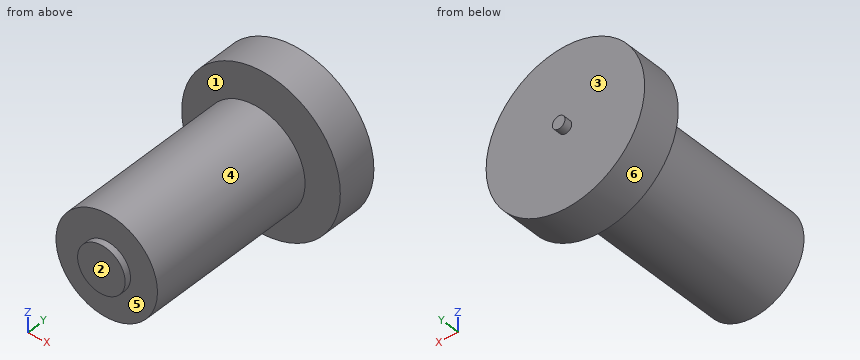
```python
from build123d import *

# Parameters (mm, degrees)
SKETCH1_R           = 32
BOSS_EXTRUDE1_DEPTH = 110
SKETCH2_R           = 5
BOSS_EXTRUDE2_DEPTH = 5
SKETCH3_R           = 50
BOSS_EXTRUDE3_DEPTH = 25
SKETCH4_R           = 4
BOSS_EXTRUDE4_DEPTH = 5
SKETCH5_R           = 15
BOSS_EXTRUDE5_DEPTH = 4


with BuildPart() as part:
    # Sketch1 → Boss-Extrude1 (new body)
    with BuildSketch(Plane(origin=(0, 0, 0), x_dir=(1, 0, 0), z_dir=(0, 1, 0))):
        Circle(SKETCH1_R)
    extrude(amount=BOSS_EXTRUDE1_DEPTH)

    # Sketch2 → Boss-Extrude2 (add)
    with BuildSketch(Plane(origin=(0, 110, 0), x_dir=(1, 0, 0), z_dir=(0, 1, 0))):
        Circle(SKETCH2_R)
    extrude(amount=BOSS_EXTRUDE2_DEPTH)

    # Sketch3 → Boss-Extrude3 (add)
    with BuildSketch(Plane(origin=(0, 115, 0), x_dir=(1, 0, 0), z_dir=(0, 1, 0))):
        Circle(SKETCH3_R)
    extrude(amount=BOSS_EXTRUDE3_DEPTH)

    # Sketch4 → Boss-Extrude4 (add)
    with BuildSketch(Plane(origin=(0, 140, 0), x_dir=(1, 0, 0), z_dir=(0, 1, 0))):
        Circle(SKETCH4_R)
    extrude(amount=BOSS_EXTRUDE4_DEPTH)

    # Sketch5 → Boss-Extrude5 (add)
    with BuildSketch(Plane.XZ):
        Circle(SKETCH5_R)
    extrude(amount=BOSS_EXTRUDE5_DEPTH)


solid = part.part
```
CAD build for the part. Positions are in the model's coordinates, mm. Face numbers are marked on the shaded views. A direction names the side the tool comes from. Coordinates: 2 decimals unless noted, no trailing zeros. Order: outer loops, then holes, each group sorted by start corner. A loop starts at its lowest first (then second) coordinate and runs counter-clockwise, first axis right, second up. Notation, with made-up numbers: M 18.5,-36.75 L 27.5,-36.75 A21 cw 27.5,-17.75 Z; hole C 78,-34.5 d2. An arc over 180 degrees is marked long. Write each question's results on one line, items separated by ' | '. Start each with the question number.
Q1. Drill centre lines: probe 1 along Y at (x, z) = (4.5, 28.5); probe 2 along Y at (x, z) = (-0.5, -43); probe 3 along Y at (x, z) = (5, -7.5). Where is each one in solid material? Low to high. Write a range as from..to.
Q2. Cut at B-B (z = 0). List the corners of the cut face in (x, y), then the cut area to 3 significant figures.
Q3. Cut at A-A (x = 12). List the corners of the cut face in (y, z).
Q4. Cut at C-C (z = 21). List the corners of the cut face in (x, y), then the cut area to 3 significant figures.
Q5. Which spindle directions (+Z, -Z, +X, -X, +Y, -Y) get a long thin tool onto all of the face, cutting with end or side? Do the marked faces 5 and 6. Say none if no direction does.
Q6. Flat gauge pins, fed straight in: P1, Ø8, axis at x = 34, z = 24, coming from the -Y side; P2, Ø1.5, axis at x = -39, z = 30, coming from the +Y side; P3, Ø3, axis at x = -0.5, z = -30, coming from the -Y side. Where does each tip first touch, or does it go through?
Q7. Cut at D-D (x = 0). List the corners of the cut face in (y, z).
Q8. Pull direction Y, two halves, no side cores. Call the marked faces 1, 2, 3 and 4: +Y half, -Y half, draft (parallel to the pull), parting line (faces both ways), or undercut.
Found:
1) probe 1: 0..110, 115..140 | probe 2: 115..140 | probe 3: -4..110, 115..140
2) outline: M -50,115 L -5,115 L -5,110 L -32,110 L -32,0 L -15,0 L -15,-4 L 15,-4 L 15,0 L 32,0 L 32,110 L 5,110 L 5,115 L 50,115 L 50,140 L 4,140 L 4,145 L -4,145 L -4,140 L -50,140 Z | area: 9,750 mm²
3) outline: M -4,-9 L 0,-9 L 0,-29.66 L 110,-29.66 L 110,29.66 L 0,29.66 L 0,9 L -4,9 Z; M 115,-48.54 L 140,-48.54 L 140,48.54 L 115,48.54 Z
4) outline: M -45.38,115 L 45.38,115 L 45.38,140 L -45.38,140 Z; M -24.15,0 L 24.15,0 L 24.15,110 L -24.15,110 Z | area: 7,580 mm²
5) face 5: -Y | face 6: +Y, -Y
6) P1: y = 115 | P2: y = 140 | P3: y = 0
7) outline: M -4,-15 L 0,-15 L 0,-32 L 110,-32 L 110,-5 L 115,-5 L 115,-50 L 140,-50 L 140,-4 L 145,-4 L 145,4 L 140,4 L 140,50 L 115,50 L 115,5 L 110,5 L 110,32 L 0,32 L 0,15 L -4,15 Z
8) face 1: undercut | face 2: -Y half | face 3: +Y half | face 4: draft
